Can you work these out from the model? Positions are in its coordinate system, mm. A direction names the side the tool comes from. Give positions to 0.01 mm unless a question says otherwise; leave off trailing zeros. Order: outer loops, then holes, each group sorted by start corner. A loop starts at its lowest first (then second) coordinate and runs counter-clockwise, first axis right, second up.
Item 1: If I drill on line 1 along X through (y, z) = (4, 30.3); line 2 along X through (y, z) = (5, 28.35); line 3 along Z through (x, y) = (-19, -0.25), over which ranges is the centre line in solid material (lowest first)?
Item 2: Which directions (+Z, -Z, +X, -X, +Y, -Y) give clear straight access to the entire face, cutting with the end or side of a thin tool? Please do faces 4 (the flat face through (-9, 1, 31.512)), 5 (the cylindrical face through (-35, 0, -3)), 6 (the flat face through (-35, 0, -5)), 7 (the flat face through (1, 6, 29.262)), 8 (the cylindrical face through (-25.457, -0.028, 25.946)).
Item 3: I want a section at A-A, the plane x = -18. Write out the boundary of the cut face in (y, z), then the cut area to 3 significant figures.
Item 4: I want a section at D-D, the plane z = 17. Write out the boundary of the cut face in (x, y), then the cut area to 3 significant figures.
Item 5: I want a section at C-C, the plane x = 0. Write out the boundary of the cut face in (y, z), then the cut area to 3 significant figures.
Item 6: If we mould it in two halves opening along Y, with no side actions, what happens to faces 1 (the flat face through (-33.356, -0.028, 1.21)), 2 (the cylindrical face through (-2.698, -1.665, 29.787)), 3 (the cylindrical face through (-0.759, 7.417, 30.403))? For each: +Y half, -Y half, draft (parallel to the pull), parting line (faces both ways), or undercut.
Item 7: I'm going to push flat-ended pins straight in: pin 1 Ø1.1 at (x, z) = (-10, 30) entering from +Y; pin 2 Ø3.5 at (x, y) = (0, 4) entering from +Z; pin 3 Ø1.5 at (y, z) = (4, 29) entering from -X. Where does each tip first touch, or does it pass through?
```python
from build123d import *

# Parameters (mm, degrees)
PAD063_DEPTH       = 2
PAD064_DEPTH       = 3.5
SKETCH106_R        = 3.5
POCKET003047_DEPTH = 2.25
SKETCH107_R        = 4.702209
PAD065_DEPTH       = 1.2
SKETCH108_R        = 1.7
POCKET003048_DEPTH = 5
PAD066_DEPTH       = 3.5
SKETCH110_R        = 1.7
POCKET003049_DEPTH = 5
POCKET003050_DEPTH = 3
PAD068_DEPTH       = 4


with BuildPart() as obj1:
    # Sketch104 → Pad063 (new body, symmetric)
    with BuildSketch(Plane.XZ):
        with BuildLine():
            Line((7.19326, 28.01235), (20.118014, 28.01235))
            ThreePointArc((27.996703, 20.985646), (25.396468, 26.000474), (20.118014, 28.01235))
            Line((27.996703, 20.985646), (30.977077, -4.999855))
            Line((33.977077, -4.999855), (30.977077, -4.999855))
            Line((31.375084, 21.001564), (33.977077, -4.999855))
            ThreePointArc((31.375084, 21.001564), (27.724482, 28.375326), (20.118014, 31.51235))
            Line((7.19326, 31.51235), (20.118014, 31.51235))
            Line((7.19326, 28.01235), (7.19326, 31.51235))
        make_face()
    extrude(amount=PAD063_DEPTH, both=True)

    # Sketch105 → Pad064 (new body)
    with BuildSketch(Plane(origin=(0, 0, 31.51235), x_dir=(-1, 0, 0), z_dir=(0, 0, 1))):
        with BuildLine():
            Line((-18, 2), (-18, -2))
            Line((-18, -2), (-4.3876, -2))
            ThreePointArc((-4.3876, -2), (1.938593, -8.415251), (1.496731, 0.583689))
            ThreePointArc((1.496731, 0.583689), (-2.758605, 1.674941), (-7.139591, 2))
            Line((-18, 2), (-7.139591, 2))
        make_face()
    extrude(amount=-PAD064_DEPTH)

    # Sketch106 → Pocket003047 (cut)
    with BuildSketch(Plane(origin=(0, 0, 31.51235), x_dir=(-1, 0, 0), z_dir=(0, 0, 1))):
        with Locations((0, -4)):
            Circle(SKETCH106_R)
    extrude(amount=-POCKET003047_DEPTH, mode=Mode.SUBTRACT)

    # Sketch107 → Pad065 (new body)
    with BuildSketch(Plane(origin=(0, 0, 28.01235), x_dir=(1, 0, 0), z_dir=(0, 0, -1))):
        with Locations((-0.089106, -3.841625)):
            Circle(SKETCH107_R)
    extrude(amount=PAD065_DEPTH)

    # Sketch108 → Pocket003048 (cut)
    with BuildSketch(Plane(origin=(0, 0, 29.26235), x_dir=(-1, 0, 0), z_dir=(0, 0, 1))):
        with Locations((-0.080471, -3.899184)):
            Circle(SKETCH108_R)
    extrude(amount=-POCKET003048_DEPTH, mode=Mode.SUBTRACT)

    # Sketch109 → Pad066 (new body)
    with BuildSketch(Plane(origin=(0, 0, 31.51235), x_dir=(-1, 0, 0), z_dir=(0, 0, 1))):
        with BuildLine():
            Line((-22.021201, -1.987049), (-22.021201, -4.986919))
            ThreePointArc((-22.021201, -4.986919), (-17.510002, -9.511218), (-12.998803, -4.986919))
            Line((-12.998803, -4.986919), (-12.998803, -1.987049))
            Line((-22.021201, -1.987049), (-12.998803, -1.987049))
        make_face()
    extrude(amount=-PAD066_DEPTH)

    # Sketch110 → Pocket003049 (cut)
    with BuildSketch(Plane(origin=(0, 0, 31.51235), x_dir=(-1, 0, 0), z_dir=(0, 0, 1))):
        with Locations((-17.491917, -5)):
            Circle(SKETCH110_R)
    extrude(amount=-POCKET003049_DEPTH, mode=Mode.SUBTRACT)

    # Sketch111 → Pocket003050 (cut)
    with BuildSketch(Plane(origin=(0, 0, 31.51235), x_dir=(-1, 0, 0), z_dir=(0, 0, 1))):
        Polygon((-14.138998, -5.003928), (-15.835596, -2.057479), (-19.235593, -2.053552), (-20.938994, -4.996072), (-19.242396, -7.942521), (-15.842399, -7.946448), align=None)
    extrude(amount=-POCKET003050_DEPTH, mode=Mode.SUBTRACT)

    # Sketch112 → Pad068 (new body)
    with BuildSketch(Plane.XZ.offset(2)):
        with BuildLine():
            Line((27, 28.536497), (32.513573, -5))
            Line((32.513573, -5), (37.000002, -5))
            Line((37.000002, -5), (37.000002, -4.583553))
            ThreePointArc((33.505627, -1), (35.019116, -3.019659), (37.000002, -4.583553))
            Line((33, 5), (33.505627, -1))
            Line((35, 3.304739), (33, 5))
            Line((32.728943, 7), (35, 3.304739))
            Line((32, 13), (32.728943, 7))
            Line((34.496559, 10.608005), (32, 13))
            Line((32, 15), (34.496559, 10.608005))
            Line((31, 20), (32, 15))
            Line((33.606815, 17.606869), (31, 20))
            Line((31, 22), (33.606815, 17.606869))
            Line((27, 28.536497), (31, 22))
        make_face()
    extrude(amount=-PAD068_DEPTH)


with BuildPart() as part_mirroring012:
    # Part__Mirroring012: instance of obj1
    add(obj1.part.mirror(Plane(origin=(0, 0, 0), x_dir=(0, -1, 0), z_dir=(1, 0, 0))))


solid = part_mirroring012.part
```
Results list:
1. line 1: x = -22.02 to -20.36, -14.72 to -13, -4.82 to -3.5, 3.5 to 4.82
1. line 2: x = -22.02 to -19.19, -15.79 to -13, -4.72 to -1.38, 1.21 to 4.72
1. line 3: z = 28.01 to 31.51
2. face 4: +Z, +X, -X, +Y, -Y
2. face 5: -X, +Y, -Y
2. face 6: -Z, +X, -X, +Y, -Y
2. face 7: +Z
2. face 8: -Z, +Y, -Y
3. outline: (-2, 28.01) - (3.38, 28.01) - (3.38, 28.51) - (2.05, 28.51) - (2.05, 31.51) - (-2, 31.51) - close; (6.62, 28.01) - (9.48, 28.01) - (9.48, 31.51) - (7.94, 31.51) - (7.94, 28.51) - (6.62, 28.51) - close
3. area: 20.9 mm2
4. outline: (-31.78, -2) - (-28.45, -2) - (-28.45, 2) - (-31.78, 2) - close
4. area: 13.3 mm2
5. outline: (-1.06, 28.01) - (-0.86, 28.01) - (-0.86, 26.81) - (2.2, 26.81) - (2.2, 29.26) - (0.5, 29.26) - (0.5, 31.51) - (-1.06, 31.51) - close; (5.6, 26.81) - (8.54, 26.81) - (8.54, 28.01) - (8.82, 28.01) - (8.82, 31.51) - (7.5, 31.51) - (7.5, 29.26) - (5.6, 29.26) - close
5. area: 21.8 mm2
6. face 1: draft
6. face 2: -Y half
6. face 3: undercut
7. pin 1: stops at y = 2
7. pin 2: stops at z = 29.26
7. pin 3: stops at x = -22.02
